Part model, mm, in its own coordinate system. A direction names the side the tool comes from. Round coordinates to 2 decimals unless told otherwise and drop trailing zeros. Write each loop counter-clockwise with the first axis right and the second up, starting at its lowest first coordinate (ties: lowest second). Pieces come first, ordered by that corner, then holes.
```python
from build123d import *

# Parameters (mm, degrees)
F0_R     = 10
F0_R_2   = 2.5
F2_DEPTH = 12.5
F3_D     = 5
F3_DEPTH = 5
F3_TIP   = 1.5021515476
F5_DEPTH = 14.868


with BuildPart() as f2:
    # F0 (on Right) → F2 (new body, symmetric)
    with BuildSketch(Plane.YZ):
        Circle(F0_R)
        Circle(F0_R_2, mode=Mode.SUBTRACT)
        Circle(F0_R_2)
    extrude(amount=F2_DEPTH, both=True)

    # F3
    with Locations(Plane.YZ.offset(12.5)):
        with Locations((0, 0)):
            Hole(F3_D / 2, depth=F3_DEPTH)
            with Locations((0, 0, -(F3_DEPTH + F3_TIP / 2))):  # 118° drill point
                Cone(0, F3_D / 2, F3_TIP, mode=Mode.SUBTRACT)

    # F4 (on face) → F5 (cut)
    with BuildSketch(Plane(origin=(-12.5, 0, 0), x_dir=(0, -1, 0), z_dir=(-1, 0, 0))):
        with BuildLine():
            Line((1.4575, 2.025023148), (-1.4575, 2.025023148))
            ThreePointArc((-1.4575, 2.025023148), (0, -2.495), (1.4575, 2.025023148))
        make_face()
    extrude(amount=-F5_DEPTH, mode=Mode.SUBTRACT)


solid = f2.part
```
Q1. Which spindle directions (+Z, -Z, +X, -X, +Y, -Y) get a long thin tool onto all of the face, cutting with end or side? Do faces 1 (the flat face through (-12.5, -0.1, 2.4)), 2 (the cylindrical face through (9.96, 0.54, -2.44)), 3 (the flat face through (-5, 0, 2.025)). Say none if no direction does.
Values follow:
face 1: +Z, -Z, -X, +Y, -Y
face 2: +X
face 3: -X
Q2. Cut at B-B on z = -3.5. Write the cut outline in (x, y), plus the area to 3 significant figures.
Values follow:
outline: (-12.5, -9.37) - (12.5, -9.37) - (12.5, 9.37) - (-12.5, 9.37) - close
area: 468 mm2
Q3. Wall check: L1, parallel to Z at x = 10.1, y = 0; L2, parallel to Y at x = -6.75, z = 0.5; L3, parallel to Z at x = 10.25, y = 2.25. Give the ranges that are in metal, low to high.
Values follow:
L1: z = -10 to -2.5, 2.5 to 10
L2: y = -9.99 to -2.44, 2.44 to 9.99
L3: z = -9.74 to -1.09, 1.09 to 9.74
Q4. Drop flat-ended pins along their axis: pin 1 (2.5 mm diameter, centred on y = 1, z = -1, fed in from -X); pin 2 (2 mm diameter, centred on x = -3, z = 8, fed in from -Y); pin 3 (2 mm diameter, centred on y = -1, z = 0, fed in from +X); pin 4 (2 mm diameter, centred on x = -3.5, z = -2.5, fed in from -Y). Give the stop position or say it passes through.
Values follow:
pin 1: stops at x = -12.5
pin 2: stops at y = -7.14
pin 3: stops at x = 7.2
pin 4: stops at y = -9.89
Q5. Cut at C-C on y = -3.25. Write the cut outline in (x, z), plus the area to 3 significant figures.
Values follow:
outline: (-12.5, -9.46) - (12.5, -9.46) - (12.5, 9.46) - (-12.5, 9.46) - close
area: 473 mm2
Q6. Cut at D-D on x = -3. Write the cut outline in (y, z) (1 decimal), plus the area to 3 significant figures.
Values follow:
outline: circle Ø20 at (0, 0); hole (-1.5, 2) arc R2.5 ccw (long way) to (1.5, 2) - close
area: 296 mm2
Q7. Cut at A-A on x = 8.75. Write the cut outline in (y, z), plus the area to 3 significant figures.
Values follow:
outline: circle Ø20 at (0, 0); hole circle Ø5 at (0, 0)
area: 295 mm2
Q8. Mould opens along Y. For faces 4 (the flat face through (2.368, 0, 0)), 5 (the flat face through (12.5, 2, -2)), 6 (the cylindrical face through (0.18, -2.17, -9.76)) say: +Y half, -Y half, draft (parallel to the pull), parting line (faces both ways), or undercut.
Values follow:
face 4: undercut
face 5: draft
face 6: parting line
